Geometry check sheet. Reference: the model listing, model coordinates, mm. A direction names the side the tool comes from. Give positions to 0.01 mm unless a question says otherwise; leave off trailing zeros. Order: outer loops, then holes, each group sorted by start corner. A loop starts at its lowest first (then second) coordinate and runs counter-clockwise, first axis right, second up. Notation, with made-up numbers: M 21.25,-33 L 49.25,-33 A25 cw 49.25,-5 Z; hole C -35,-18 d4. An arc over 180 degrees is marked long. Answer as CSV lines item,"result".
from build123d import *

# Parameters (mm, degrees)
SKETCH1_R           = 3.5
SKETCH1_R_2         = 6
SKETCH1_R_3         = 2.5
SKETCH1_R_4         = 2
SKETCH1_R_5         = 10.5
BOSS_EXTRUDE1_DEPTH = 5
FILLET2_R           = 15


with BuildPart() as part:
    # Sketch1 → Boss-Extrude1 (new body)
    with BuildSketch(Plane(origin=(0, 0, 0), x_dir=(1, 0, 0), z_dir=(0, 1, 0))):
        with BuildLine():
            Line((40, -25), (40, -35))
            Line((40, -35), (90, -35))
            Line((90, -35), (90, 35))
            Line((90, 35), (40, 35))
            Line((40, 35), (40, 25))
            Line((40, 25), (0, 25))
            ThreePointArc((0, 25), (-25, 0), (0, -25))
            Line((0, -25), (40, -25))
        make_face()
        with Locations(Location((65, 24, 0), (0, 0, 270))):
            Circle(SKETCH1_R, mode=Mode.SUBTRACT)
        with Locations(Location((65, -24, 0), (0, 0, 270))):
            Circle(SKETCH1_R, mode=Mode.SUBTRACT)
        with Locations(Location((65, 0, 0), (0, 0, 270))):
            Circle(SKETCH1_R_2, mode=Mode.SUBTRACT)
        with Locations(Location((35, 0, 0), (0, 0, 270))):
            Circle(SKETCH1_R_3, mode=Mode.SUBTRACT)
        with Locations(Location((0, -15, 0), (0, 0, 270))):
            Circle(SKETCH1_R_4, mode=Mode.SUBTRACT)
        with Locations(Location((-12.990381057, -7.5, 0), (0, 0, 270))):
            Circle(SKETCH1_R_4, mode=Mode.SUBTRACT)
        with Locations(Location((12.990381057, -7.5, 0), (0, 0, 270))):
            Circle(SKETCH1_R_4, mode=Mode.SUBTRACT)
        with Locations(Location((-12.990381057, 7.5, 0), (0, 0, 270))):
            Circle(SKETCH1_R_4, mode=Mode.SUBTRACT)
        with Locations(Location((0, 0, 0), (0, 0, 270))):
            Circle(SKETCH1_R_5, mode=Mode.SUBTRACT)
        with Locations(Location((0, 15, 0), (0, 0, 270))):
            Circle(SKETCH1_R_4, mode=Mode.SUBTRACT)
        with Locations(Location((12.990381057, 7.5, 0), (0, 0, 270))):
            Circle(SKETCH1_R_4, mode=Mode.SUBTRACT)
    extrude(amount=BOSS_EXTRUDE1_DEPTH)

    # Fillet2
    # the kernel refuses this fillet: 15 mm, written as the material it takes off along each edge
    with BuildSketch(Plane(origin=(40, -35.355339059, -35), x_dir=(1, 0, 0), z_dir=(0, 1, 0))) as fillet2_piece_1:
        with BuildLine():
            CenterArc((14.142135624, -15), FILLET2_R, 90, 70.528779366)
            Line((0, -10), (-0.282842712, -9.9))
            ThreePointArc((-0.282842712, -9.9), (-0.3, -5), (-0.3, 0))
            Line((-0.3, 0), (0, 0.3))
            Line((0, 0.3), (14.142135624, 0.3))
            Line((14.142135624, 0.3), (14.142135624, 0))
        make_face()
    extrude(amount=75.710678119, mode=Mode.SUBTRACT)
    with BuildSketch(Plane(origin=(90, -37.5, 35), x_dir=(-1, 0, 0), z_dir=(0, 1, 0)), Plane(origin=(90, -37.5, -35), x_dir=(0, 0, 1), z_dir=(0, 1, 0))) as fillet2_piece_2:
        with BuildLine():
            CenterArc((FILLET2_R, -FILLET2_R), FILLET2_R, 90, 90)
            Line((0, -FILLET2_R), (-FILLET2_R * 0.02, -FILLET2_R))
            Line((-FILLET2_R * 0.02, -FILLET2_R), (-FILLET2_R * 0.02, FILLET2_R * 0.02))
            Line((-FILLET2_R * 0.02, FILLET2_R * 0.02), (FILLET2_R, FILLET2_R * 0.02))
            Line((FILLET2_R, FILLET2_R * 0.02), (FILLET2_R, 0))
        make_face()
    extrude(amount=80, mode=Mode.SUBTRACT)
    with BuildSketch(Plane(origin=(40, -35.355339059, 35), x_dir=(0, 0, -1), z_dir=(0, 1, 0))) as fillet2_piece_3:
        with BuildLine():
            CenterArc((15, -14.142135624), FILLET2_R, 109.471220634, 70.528779366)
            Line((0, -14.142135624), (-0.3, -14.142135624))
            Line((-0.3, -14.142135624), (-0.3, 0))
            Line((-0.3, 0), (0, 0.3))
            ThreePointArc((0, 0.3), (5, 0.3), (9.9, 0.282842712))
            Line((9.9, 0.282842712), (10, 0))
        make_face()
    extrude(amount=75.710678119, mode=Mode.SUBTRACT)


solid = part.part
(1) Section check B-B on z = 0. Enter the section's corners in (x, y).
The answers:
outline,"M -25,0 L -10.5,0 L -10.5,5 L -25,5 Z; M 10.5,0 L 32.5,0 L 32.5,5 L 10.5,5 Z; M 37.5,0 L 59,0 L 59,5 L 37.5,5 Z; M 71,0 L 90,0 L 90,5 L 71,5 Z"
(2) Material ranges on line 1 (X direction, y = 2.65, z = 0); line 2 (X direction, y = 2.7, z = -4); line 3 (X direction, y = 3.05, z = 5), recorded low to high.
The answers:
line 1,"x = -25 to -10.5, 10.5 to 32.5, 37.5 to 59, 71 to 90"
line 2,"x = -24.68 to -9.71, 9.71 to 60.53, 69.47 to 90"
line 3,"x = -24.49 to -9.23, 9.23 to 61.68, 68.32 to 90"
(3) Gauge pin test, flat ends, axial feed: P1, Ø1.5, axis at y = 4, z = 3, coming from the -X side; P2, Ø1.5, axis at x = 18, y = 3, coming from the +Z side; P3, Ø1.5, axis at y = 1.5, z = -25.5, coming from the +X side. Record the tip position at first contact, or that the pin passes through.
The answers:
P1,"stops at x = -24.9"
P2,"stops at z = 25"
P3,"stops at x = 89.23"
(4) Section check D-D on y = 2.05. State how many separate pieces and enclosed holes the cut face has, then the cut area to 3 significant figures.
The answers:
separate pieces,"1"
enclosed holes,"11"
area,"5,680 mm2"
(5) Draft check along Z on faces 1 (the face through (64, 2, 35)), 2 (the face through (85.72, 2.47, -30.49)), 3 (the face through (67.95, 2.46, 25.88)), 4 (the face through (3.2, 2.5, 10)). Enter one of: +Z half, -Z half, draft (parallel to the pull), parting line (faces both ways), or undercut.
The answers:
face 1,"+Z half"
face 2,"-Z half"
face 3,"undercut"
face 4,"undercut"
(6) Section check A-A on z = 15. Enter the section's corners in (x, y).
The answers:
outline,"M -20,0 L -2,0 L -2,5 L -20,5 Z; M 2,0 L 90,0 L 90,5 L 2,5 Z"
(7) Section check C-C on x = -4.5. Enter the section's corners in (y, z), then the cut area to 3 significant figures.
The answers:
outline,"M 0,-24.59 L 5,-24.59 L 5,-9.49 L 0,-9.49 Z; M 0,9.49 L 5,9.49 L 5,24.59 L 0,24.59 Z"
area,"151 mm2"
(8) Tool access check on faces 5 (the face through (20, 2, -25)), 6 (the face through (14.342, 2.465, -8.974)). Record the directions out of +Z, -Z, +X, -X, +Y, -Y that give a thin tool (end or side, any length) a straight path to the whole face; none if there is none.
The answers:
face 5,"-Z, -X, +Y, -Y"
face 6,"+Y, -Y"
